```python
from build123d import *

# Parameters (mm, degrees)
BOSS_EXTRU_1_DEPTH = 4.900038


with BuildPart() as part:
    # Esquisse1 → Boss.-Extru.1 (new body)
    with BuildSketch(Plane(origin=(0, 4.900038, 0), x_dir=(1, 0, 0), z_dir=(0, 1, 0))):
        with BuildLine():
            Line((20.352144301, -2.543463741), (20.352144301, -2.043462703))
            Line((20.352144301, -2.043462703), (20.222233634, -1.234634479))
            Line((20.222233634, -1.234634479), (19.788693601, -0.58578943))
            Line((19.788693601, -0.58578943), (19.139843552, -0.152243798))
            Line((19.139843552, -0.152243798), (18.374483494, -2.386e-06))
            Line((18.374483494, -2.386e-06), (13.150843099, -2.386e-06))
            Line((13.150843099, -2.386e-06), (12.570463055, -0.086064053))
            Line((12.570463055, -0.086064053), (12.040033015, -0.336843111))
            Line((12.040033015, -0.336843111), (10.798452921, -1.006549462))
            Line((10.798452921, -1.006549462), (9.453426819, -1.431914494))
            Line((9.453426819, -1.431914494), (8.640349758, -1.813265523))
            Line((8.640349758, -1.813265523), (8.076110715, -2.511950576))
            Line((8.076110715, -2.511950576), (7.8744797, -3.387092642))
            Line((7.8744797, -3.387092642), (7.8744797, -24.738594256))
            Line((7.8744797, -24.738594256), (7.650796683, -25.657674326))
            Line((7.650796683, -25.657674326), (7.029780636, -26.37116438))
            Line((7.029780636, -26.37116438), (6.15034157, -26.719484406))
            Line((6.15034157, -26.719484406), (4.29809943, -27.122544437))
            Line((4.29809943, -27.122544437), (2.528101296, -27.801054488))
            Line((2.528101296, -27.801054488), (0.881055671, -28.739404559))
            Line((0.881055671, -28.739404559), (0.280930026, -29.374954607))
            Line((0.280930026, -29.374954607), (0.009177495, -30.20574467))
            Line((0.009177495, -30.20574467), (0.117708214, -31.073094735))
            Line((0.117708214, -31.073094735), (0.585789149, -31.811314791))
            Line((0.585789149, -31.811314791), (2.228685273, -33.454204915))
            Line((2.228685273, -33.454204915), (2.442788289, -33.580814925))
            Line((2.442788289, -33.580814925), (2.691403308, -33.588594925))
            Line((2.691403308, -33.588594925), (2.913002325, -33.475614917))
            ThreePointArc((2.913002325, -33.475614917), (13.213872644, -33.833045583), (13.430577738, -44.137836939))
            Line((13.430577738, -44.137836939), (13.363553773, -44.3265459))
            Line((13.363553773, -44.3265459), (13.371323773, -44.575155919))
            Line((13.371323773, -44.575155919), (13.497933783, -44.789265935))
            Line((13.497933783, -44.789265935), (15.140833907, -46.432156059))
            Line((15.140833907, -46.432156059), (15.879053963, -46.900236095))
            Line((15.879053963, -46.900236095), (16.746394029, -47.008766103))
            Line((16.746394029, -47.008766103), (17.577194091, -46.737016082))
            Line((17.577194091, -46.737016082), (18.212744139, -46.136886037))
            Line((18.212744139, -46.136886037), (19.385584228, -43.963185873))
            Line((19.385584228, -43.963185873), (20.108124283, -41.601305694))
            Line((20.108124283, -41.601305694), (20.352144301, -39.143465508))
            Line((20.352144301, -39.143465508), (20.352144301, -30.743464873))
            Line((20.352144301, -30.743464873), (20.285154296, -30.493464854))
            Line((20.285154296, -30.493464854), (20.102144282, -30.31045484))
            Line((20.102144282, -30.31045484), (19.852144263, -30.243464835))
            Line((19.852144263, -30.243464835), (16.602144018, -30.243464835))
            Line((16.602144018, -30.243464835), (16.568644015, -30.368465215))
            Line((16.568644015, -30.368465215), (16.477144008, -30.459975222))
            Line((16.477144008, -30.459975222), (16.352143999, -30.493465225))
            Line((16.352143999, -30.493465225), (16.227143989, -30.459975222))
            Line((16.227143989, -30.459975222), (16.135633982, -30.368465215))
            Line((16.135633982, -30.368465215), (16.10214398, -30.243465206))
            Line((16.10214398, -30.243465206), (16.135633982, -30.118465196))
            Line((16.135633982, -30.118465196), (16.227143989, -30.026955189))
            Line((16.227143989, -30.026955189), (16.352143999, -29.993465187))
            Line((16.352143999, -29.993465187), (16.352143999, -25.593464854))
            Line((16.352143999, -25.593464854), (16.227143989, -25.559974852))
            Line((16.227143989, -25.559974852), (16.135633982, -25.468464845))
            Line((16.135633982, -25.468464845), (16.10214398, -25.343464835))
            Line((16.10214398, -25.343464835), (16.135633982, -25.218464826))
            Line((16.135633982, -25.218464826), (16.227143989, -25.126954819))
            Line((16.227143989, -25.126954819), (16.352143999, -25.093464816))
            Line((16.352143999, -25.093464816), (16.477144008, -25.126954819))
            Line((16.477144008, -25.126954819), (16.568644015, -25.218464826))
            Line((16.568644015, -25.218464826), (16.602144018, -25.343464835))
            Line((16.602144018, -25.343464835), (27.852144868, -25.343464835))
            ThreePointArc((27.852144868, -25.343464835), (28.205698285, -25.197018215), (28.352144906, -24.843464798))
            Line((28.352144906, -24.843464798), (28.352144906, -8.443464873))
            ThreePointArc((28.352144906, -8.443464873), (28.205698285, -8.089911456), (27.852144868, -7.943464835))
            Line((27.852144868, -7.943464835), (16.602144018, -7.943464835))
            Line((16.602144018, -7.943464835), (16.568644015, -8.068465529))
            Line((16.568644015, -8.068465529), (16.477144008, -8.159969536))
            Line((16.477144008, -8.159969536), (16.352143999, -8.193464539))
            Line((16.352143999, -8.193464539), (16.227143989, -8.159969536))
            Line((16.227143989, -8.159969536), (16.135633982, -8.068465529))
            Line((16.135633982, -8.068465529), (16.10214398, -7.94346352))
            Line((16.10214398, -7.94346352), (16.135633982, -7.81846451))
            Line((16.135633982, -7.81846451), (16.227143989, -7.726956504))
            Line((16.227143989, -7.726956504), (16.352143999, -7.693462501))
            Line((16.352143999, -7.693462501), (16.352143999, -3.293462168))
            Line((16.352143999, -3.293462168), (16.227143989, -3.259968166))
            Line((16.227143989, -3.259968166), (16.135633982, -3.168464159))
            Line((16.135633982, -3.168464159), (16.10214398, -3.043462149))
            Line((16.10214398, -3.043462149), (16.135633982, -2.91846314))
            Line((16.135633982, -2.91846314), (16.227143989, -2.826955133))
            Line((16.227143989, -2.826955133), (16.352143999, -2.793465131))
            Line((16.352143999, -2.793465131), (16.477144008, -2.826955133))
            Line((16.477144008, -2.826955133), (16.568644015, -2.91846314))
            Line((16.568644015, -2.91846314), (16.602144018, -3.043464835))
            Line((16.602144018, -3.043464835), (19.852144263, -3.043464835))
            Line((19.852144263, -3.043464835), (20.102144282, -2.97647983))
            Line((20.102144282, -2.97647983), (20.285154296, -2.793467816))
            Line((20.285154296, -2.793467816), (20.352144301, -2.543463741))
        make_face()
    extrude(amount=-BOSS_EXTRU_1_DEPTH)


solid = part.part
```
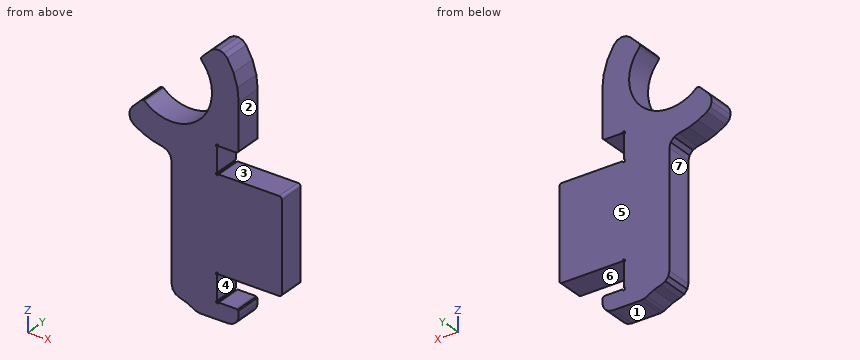
Geometry: final body of the model. Coordinates: model frame, mm. Face numbers are marked on the shaded views. A direction names the side the tool comes from. Coordinates: 2 decimals unless noted, no trailing zeros. Order: outer loops, then holes, each group sorted by start corner. A loop starts at its lowest first (then second) coordinate and runs counter-clockwise, first axis right, second up. Notation, with made-up numbers: (40, 47.5) - (93, 47.5) arc R24 cw to (93, 68.5) - close; hole circle Ø10 at (68, -12). An arc over 180 degrees is marked (long way). Return JSON: item names as keys, results as strings. Group by question number.
1. Pin query (flat end, axial travel): pin 1 (1.5 mm diameter, centred on x = 20, y = 1, fed in from +Z); pin 2 (2 mm diameter, centred on x = 14, z = 10.5, fed in from -Y); pin 3 (2.5 mm diameter, centred on y = 3, z = 35, fed in from +X); pin 4 (1.5 mm diameter, centred on y = 3.5, z = 11, fed in from -X). Return the tip coordinate at first contact, or that it passes through.
2. Material intervals for line 1 along Z through (x, y) = (16.75, 0.6); line 2 along X through (y, z) = (2.2, 13); line 3 along Z through (x, y) = (20.5, 4.65), sorted ascending. Write a range as [from, to].
3. Set-up query: the marked faces 5, 6 and 7. Return all of +Z, -Z, +X, -X, +Y, -Y with unobstructed straight access to the full face (end or side cutting, diameter ignored); none if empty.
4. Cut plane A-A (z = 5). Output: boundary loops of the cut face in (x, y).
5. Pull-direction query (Z, two-part tool) for the marked faces 1, 2, 3 and 4; classes: pulls with the +Z half, pulls with the -Z half, needs draft (parallel to the pull), parting line crosses it, or undercut.
6. Cut plane B-B (z = 19). Output: boundary loops of the cut face in (x, y).
Resolved:
{
 "1": {"pin 1": "stops at z = 44.21", "pin 2": "stops at y = 0", "pin 3": "stops at x = 20.35", "pin 4": "stops at x = 7.87"},
 "2": {"line 1": "z = [0, 3.04], [7.94, 25.34], [30.24, 47.01]", "line 2": "x = [7.87, 28.35]", "line 3": "z = [7.94, 25.34]"},
 "3": {"face 5": "+Z, -Z, +X, -X, +Y", "face 6": "+X, +Y, -Y", "face 7": "-Z, -X, +Y, -Y"},
 "4": {"outline": "(7.87, 0) - (16.35, 0) - (16.35, 4.9) - (7.87, 4.9) - close"},
 "5": {"face 1": "pulls with the -Z half", "face 2": "needs draft", "face 3": "undercut", "face 4": "undercut"},
 "6": {"outline": "(7.87, 0) - (28.35, 0) - (28.35, 4.9) - (7.87, 4.9) - close"}
}
